The model under review builds one solid part; all positions refer to its coordinate system, in mm. Face numbers are marked on the shaded views. A direction names the side the tool comes from. Give positions to 0.01 mm unless a question says otherwise; leave off trailing zeros. Order: outer loops, then holes, each group sorted by start corner. A loop starts at its lowest first (then second) coordinate and runs counter-clockwise, first axis right, second up.
```python
from build123d import *

# Parameters (mm, degrees)
BOSS_EXTRUDE1_DEPTH = 101.6
SKETCH2_R           = 14.2875
CUT_EXTRUDE1_DEPTH  = 50.8


with BuildPart() as part:
    # Sketch1 → Boss-Extrude1 (new body)
    with BuildSketch(Plane(origin=(0, 0, 0), x_dir=(-1, 0, 0), z_dir=(0, 0, -1))):
        with BuildLine():
            Line((-12.7, 25.146), (-12.7, -25.146))
            ThreePointArc((-12.7, -25.146), (-12.625605122, -25.325605122), (-12.446, -25.4))
            Line((-12.446, -25.4), (12.446, -25.4))
            ThreePointArc((12.446, -25.4), (12.625605122, -25.325605122), (12.7, -25.146))
            Line((12.7, -25.146), (12.7, 25.146))
            ThreePointArc((12.7, 25.146), (12.625605122, 25.325605122), (12.446, 25.4))
            Line((12.446, 25.4), (-12.446, 25.4))
            ThreePointArc((-12.446, 25.4), (-12.625605122, 25.325605122), (-12.7, 25.146))
        make_face()
        with BuildLine():
            Line((-11.1125, -22.225), (-11.1125, 22.225))
            ThreePointArc((-11.1125, 22.225), (-10.647532015, 23.347532015), (-9.525, 23.8125))
            Line((-9.525, 23.8125), (9.525, 23.8125))
            ThreePointArc((9.525, 23.8125), (10.647532015, 23.347532015), (11.1125, 22.225))
            Line((11.1125, 22.225), (11.1125, -22.225))
            ThreePointArc((11.1125, -22.225), (10.647532015, -23.347532015), (9.525, -23.8125))
            Line((9.525, -23.8125), (-9.525, -23.8125))
            ThreePointArc((-9.525, -23.8125), (-10.647532015, -23.347532015), (-11.1125, -22.225))
        make_face(mode=Mode.SUBTRACT)
    extrude(amount=-BOSS_EXTRUDE1_DEPTH)

    # Sketch2 → Cut-Extrude1 (cut)
    with BuildSketch(Plane.ZY.offset(12.7)):
        with Locations((25.4, 0)):
            Circle(SKETCH2_R)
    extrude(amount=-CUT_EXTRUDE1_DEPTH, mode=Mode.SUBTRACT)


solid = part.part
```
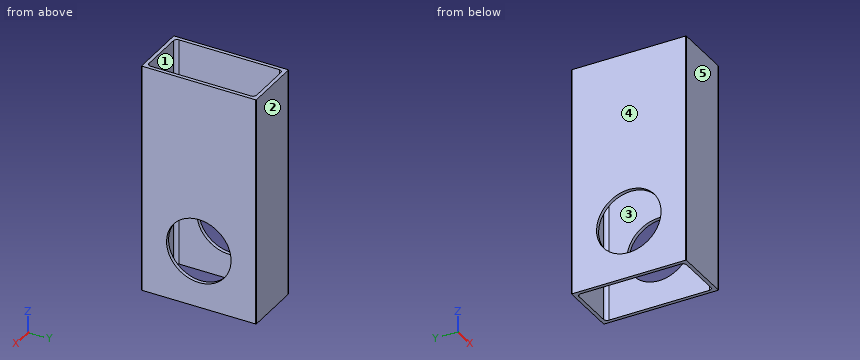
Item 1: Draft analysis for pull direction X (two halves, no side actions). For the marked faces 3, 4 and 5, state which applies: released by +X, released by -X, zero draft, split by the parting line, or undercut.
Values found:
face 3: undercut
face 4: released by -X
face 5: zero draft
Item 2: Clearance check with a flat-ended pin moving along its axis: pin 1 Ø4 at (x, y) = (-8, -9.5) entering from +Z. State where the tip first meets the part, or that it passes through.
Values found:
pin 1: passes through
Item 3: For the marked faces 1 and 2, list the 3-axis set-ups (+Z, -Z, +X, -X, +Y, -Y) from which the entire face can be reached by the end or side of a thin tool; tool diameter is ignored.
Values found:
face 1: +Z, -Z
face 2: +Z, -Z, +X, -X, +Y
Item 4: Take a section at D-D (y = 19). Give the boundary of the cut face in (x, z), and give its area (3 significant figures).
Values found:
outline: (-12.7, 0) - (-11.11, 0) - (-11.11, 101.6) - (-12.7, 101.6) - close; (11.11, 0) - (12.7, 0) - (12.7, 101.6) - (11.11, 101.6) - close
area: 323 mm2
Item 5: Take a section at B-B (y = 0). Give the boundary of the cut face in (x, z), and give its area (3 significant figures).
Values found:
outline: (-12.7, 0) - (-11.11, 0) - (-11.11, 11.11) - (-12.7, 11.11) - close; (-12.7, 39.69) - (-11.11, 39.69) - (-11.11, 101.6) - (-12.7, 101.6) - close; (11.11, 0) - (12.7, 0) - (12.7, 11.11) - (11.11, 11.11) - close; (11.11, 39.69) - (12.7, 39.69) - (12.7, 101.6) - (11.11, 101.6) - close
area: 232 mm2
Item 6: Take a section at A-A (x = 6.25). Give the boundary of the cut face in (y, z), and give its area (3 significant figures).
Values found:
outline: (-25.4, 0) - (-23.81, 0) - (-23.81, 101.6) - (-25.4, 101.6) - close; (23.81, 0) - (25.4, 0) - (25.4, 101.6) - (23.81, 101.6) - close
area: 323 mm2
Item 7: For line 1 (X direction, y = 15, z = 18.5); line 2 (Y direction, x = 12.3, z = 25.4); line 3 (Y direction, x = -5.75, z = 53), list the stretches that pass through material, from the lowest coordinate up.
Values found:
line 1: x = -12.7 to -11.11, 11.11 to 12.7
line 2: y = -25.4 to -14.29, 14.29 to 25.4
line 3: y = -25.4 to -23.81, 23.81 to 25.4
